Here's the drawing with two shaded views (mm, measured from the low corner). I have some questions. Round coordinates to 2 decimals unless told otherwise and drop trailing zeros. Order: outer loops, then holes, each group sorted by start corner. A loop starts at its lowest first (then second) coordinate and runs counter-clockwise, first axis right, second up. Notation, with made-up numbers: M 87.25,54 L 103.25,54 A9 cw 103.25,63 Z; hole C -31.75,82 d7. An arc over 180 degrees is marked long. One line per question, with ' | ' between items.
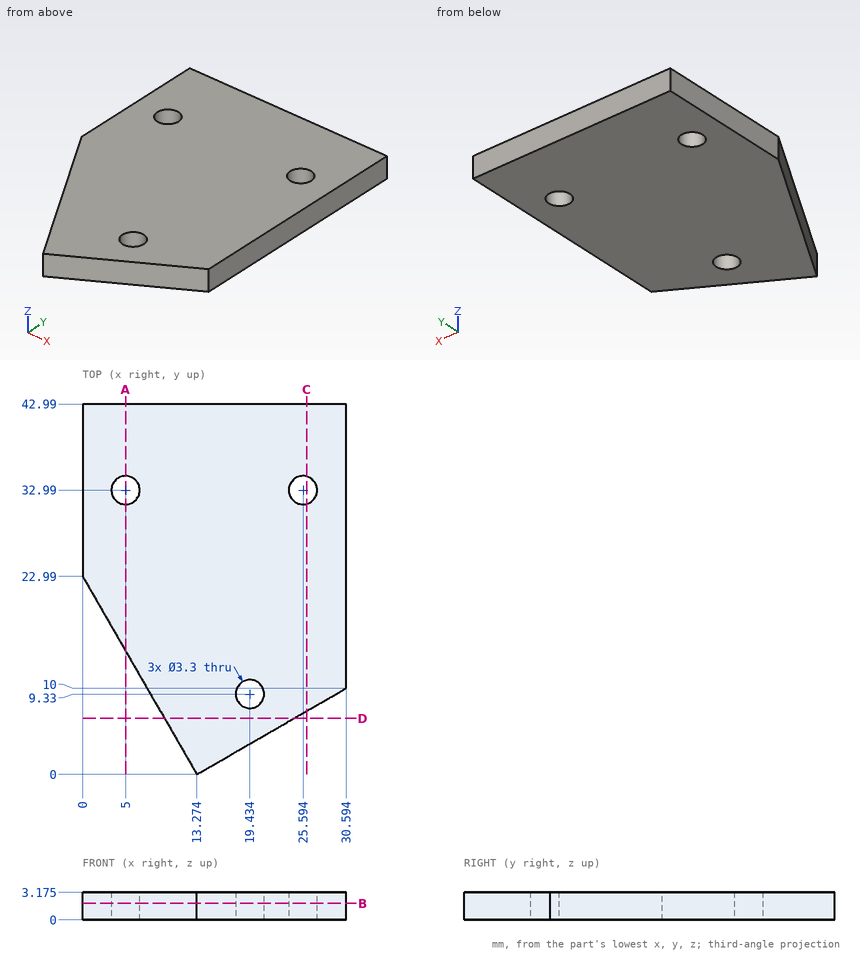
(1) If we section it at D-D on y = 6.5: Please give me the cut outline in (x, z) (1 decimal).
Final values:
outline: M 9.5,0 L 24.5,0 L 24.5,3.2 L 9.5,3.2 Z
(2) Will these pins go through, and if not, where does the flat tip stop? pin 1 Ø1 at (x, z) = (16, 1.5) entering from -Y (1 decimal); pin 2 Ø1.5 at (y, z) = (12.5, 1.5) entering from -X (1 decimal).
Final values:
pin 1: y = 1.3 | pin 2: x = 5.6
(3) If we section it at A-A on x = 5: Please give me the cut outline in (y, z) (1 decimal).
Final values:
outline: M 14.3,0 L 31.3,0 L 31.3,3.2 L 14.3,3.2 Z; M 34.6,0 L 43,0 L 43,3.2 L 34.6,3.2 Z
(4) Please list where these lines run through material, in increasing order: probe 1 along X at (y, z) = (8, 1.8) (1 decimal); probe 2 along Y at (x, z) = (18.5, 1.1); probe 3 along Y at (x, z) = (20, 2.4) (1 decimal). Write a range as [from, to].
Final values:
probe 1: [8.7, 18.5], [20.4, 27.1] | probe 2: [3.02, 7.97], [10.69, 42.99] | probe 3: [3.9, 7.8], [10.9, 43]
(5) If we section it at C-C on x = 26: Please give me the cut outline in (y, z) (1 decimal).
Final values:
outline: M 7.3,0 L 31.4,0 L 31.4,3.2 L 7.3,3.2 Z; M 34.6,0 L 43,0 L 43,3.2 L 34.6,3.2 Z
(6) If we section it at B-B on z = 1.9: State how many separate pieces and enclosed holes the cut face has, plus the area to 3 significant figures.
Final values:
separate pieces: 1 | enclosed holes: 3 | area: 1,050 mm^2
